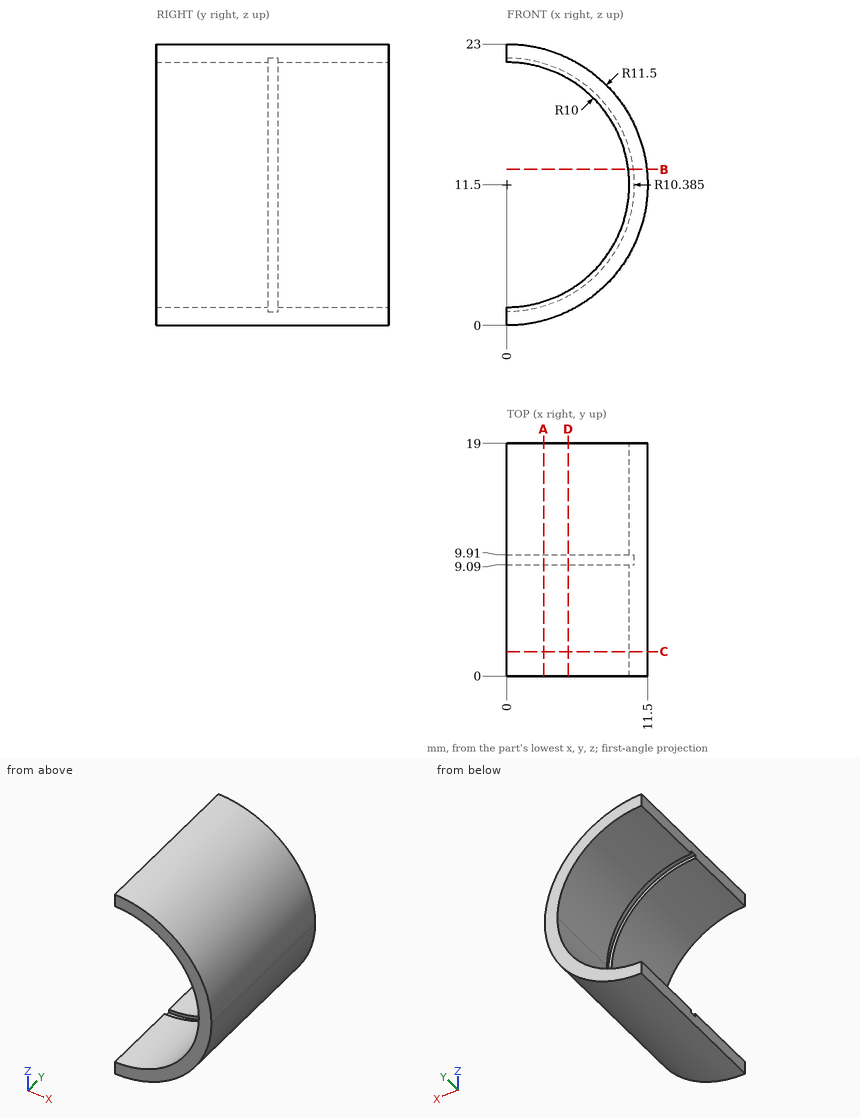
For this review, use the dimensioned drawing (mm, ordinates from the lowest corner) and the shaded views. Round coordinates to 2 decimals unless told otherwise and drop trailing zeros. Write each loop counter-clockwise with the first axis right and the second up, starting at its lowest first coordinate (ties: lowest second). Pieces come first, ordered by that corner, then holes. Notation, with made-up numbers: M -10.75,-36 L -2.75,-36 A7 ccw -2.75,-31 Z; hole C -7,-17 d7. An arc over 180 degrees is marked long. Answer as CSV lines item,"result". Start each with the question number.
Q1. Clearance check with flat-ended pins moving along their axes: P1, Ø1, axis at x = 8.5, z = 15.5, coming from the +Y side; P2, Ø10, axis at y = 16.5, z = 12.5, coming from the -X side; P3, Ø6, axis at x = 3.5, y = 12.5, coming from the +Z side; P4, Ø2, axis at x = 7.5, y = 12.5, coming from the -Z side. State where each tip first meets the part, or that it passes through.
Q2. Wall thickness on line 1 along Z through (x, y) = (1.25, 14.75); line 2 along Z through (x, y) = (6, 12); line 3 along X through (y, z) = (10.5, 20.75): over which ranges is each line inside the solid? List them lowest first.
Q3. Consider section B-B, the plane z = 12.75. Give the boundary of the cut face in (x, y).
Q4. Consider section D-D, the plane x = 5. Give the boundary of the cut face in (y, z).
Q5. Consider section A-A, the plane x = 3. Give the boundary of the cut face in (y, z), then the cut area to 3 significant figures.
Q6. Consider section C-C, the plane y = 2. Give the boundary of the cut face in (x, z), then the cut area to 3 significant figures.
Result set:
1,P1,"passes through"
1,P2,"stops at x = 8"
1,P3,"stops at z = 22.99"
1,P4,"stops at z = 2.01"
2,line 1,"z = 0.07 to 1.58, 21.42 to 22.93"
2,line 2,"z = 1.69 to 3.5, 19.5 to 21.31"
2,line 3,"x = 3.8 to 6.83"
3,outline,"M 9.92,0 L 11.43,0 L 11.43,19 L 9.92,19 L 9.92,9.91 L 10.31,9.91 L 10.31,9.09 L 9.92,9.09 Z"
4,outline,"M 0,1.14 L 19,1.14 L 19,2.84 L 9.91,2.84 L 9.91,2.4 L 9.09,2.4 L 9.09,2.84 L 0,2.84 Z; M 0,20.16 L 9.09,20.16 L 9.09,20.6 L 9.91,20.6 L 9.91,20.16 L 19,20.16 L 19,21.86 L 0,21.86 Z"
5,outline,"M 0,0.4 L 19,0.4 L 19,1.96 L 9.91,1.96 L 9.91,1.56 L 9.09,1.56 L 9.09,1.96 L 0,1.96 Z; M 0,21.04 L 9.09,21.04 L 9.09,21.44 L 9.91,21.44 L 9.91,21.04 L 19,21.04 L 19,22.6 L 0,22.6 Z"
5,area,"58.7 mm²"
6,outline,"M 0,0 A11.5 ccw 0,23 L 0,21.5 A10 cw 0,1.5 Z"
6,area,"50.7 mm²"
